The listing builds one solid part. Answer for the finished solid, in the listing's coordinates (mm). Face numbers are marked on the shaded views. A direction names the side the tool comes from. Give positions to 0.01 mm unless a question says otherwise; leave off trailing zeros. Write each loop counter-clockwise with the first axis right and the second up, starting at its lowest first coordinate (ties: lowest second). Pieces come first, ordered by that corner, then holes. Notation, with made-up numbers: (33, 1) -> (43, 1) arc R27 ccw to (43, 17) -> close; hole circle Ø8 at (-15, 76). An arc over 180 degrees is marked (long way). Write each question's results on one line, items separated by ' | '. Start each with the question number.
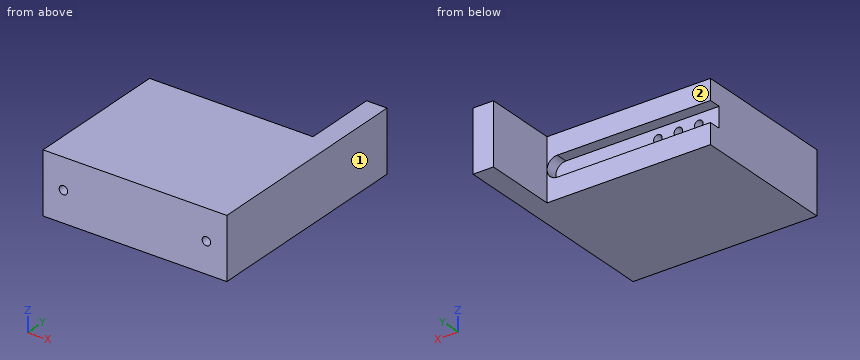
Autodesk Inventor part; units mm, degrees
ref_plane "YZ Plane" through (0, 0, 0) normal (1, 0, 0) x (0, 1, 0)
ref_plane "XZ Plane" through (0, 0, 0) normal (0, 1, 0) x (-1, 0, 0)
ref_plane "XY Plane" through (0, 0, 0) normal (0, 0, 1) x (1, 0, 0)
sketch "Sketch1" plane through (0, 0, 0) normal (0, 0, 1) x (1, 0, 0)
  line L0 (0, 0) -> (57.15, 0)
  line L1 (57.15, 0) -> (57.15, 68.2498)
  line L2 (57.15, 68.2498) -> (0, 68.2498)
  line L3 (0, 68.2498) -> (0, 0)
  line L4 (0, 68.2498) -> (50.8, 68.2498)
  line L5 (50.8, 68.2498) -> (50.8, 45.3898)
  line L6 (50.8, 45.3898) -> (0, 45.3898)
  line L7 (0, 45.3898) -> (0, 68.2498)
  dimension "d0" = 57.15
  dimension "d1" = 68.2498
  dimension "d2" = 50.8
  dimension "d3" = 22.86
extrude "Extrusion1" add sketch "Sketch1" along normal blind 19.05 contours L3 L6 L5 L2 L1 L0
sketch "Sketch2" plane through (0, 45.3898, 0) normal (0, 1, 0) x (1, 0, 0)
  line L0 (0, 0) -> (0, -19.05)
  line L1 (0, -6.35) -> (47.625, -6.35)
  line L2 (47.625, -6.35) -> (47.625, -12.7)
  line L3 (47.625, -12.7) -> (0, -12.7)
  line L4 (0, -12.7) -> (0, -6.35)
  line L5 (0, 0) -> (50.8, 0)
  circle A0 centre (47.625, -9.525) radius 3.175
  dimension "d6" = 47.625
  dimension "d7" = 6.35
  dimension "d8" = 6.35
extrude "Extrusion2" cut sketch "Sketch2" against normal blind 3.7084
sketch "Sketch3" plane through (0, 41.6814, 0) normal (0, 1, 0) x (1, 0, 0)
  line L0 (47.625, -12.7) -> (0, -12.7)
  line L1 (0, -6.35) -> (47.625, -6.35)
  line L2 (0, -12.7) -> (0, -6.35)
  point P0 (0, 0)
  point P1 (6.35, -9.525)
  point P2 (12.7, -9.525)
  point P3 (19.05, -9.525)
  dimension "d11" = 6.35
  dimension "d12" = 3.175
  dimension "d13" = 3.175
  dimension "d14" = 3.175
  dimension "d15" = 6.35
  dimension "d16" = 12.7
  dimension "d17" = 19.05
sketch "Sketch4" plane through (0, 0, 0) normal (0, -1, 0) x (1, 0, 0)
  line L0 (0, 0) -> (57.15, 0)
  line L1 (0, 19.05) -> (57.15, 19.05)
  line L2 (0, 0) -> (0, 19.05)
  line L3 (57.15, 0) -> (57.15, 19.05)
  point P0 (6.35, 9.525)
  point P1 (50.8, 9.525)
  dimension "d18" = 19.05
  dimension "d19" = 9.525
  dimension "d20" = 9.525
  dimension "d21" = 6.35
  dimension "d22" = 6.35
hole "Hole1" at (50.8, 0, 9.525) at (6.35, 0, 9.525) direction (0, 1, 0) diameter 2.6416 depth 7.112 tip angle 118
hole "Hole2" at (6.35, 41.6814, 9.525) at (12.7, 41.6814, 9.525) at (19.05, 41.6814, 9.525) direction (0, -1, 0) diameter 2.6416 depth 7.112 tip angle 118
equation "\"d8\" = d7"
properties part number "Spring block"
1. Section A-A (x = 35.5) is taken. Write down the section's boundary in (y, z), then the cut area to 3 significant figures.
2. Section C-C (y = 54) is taken. Write down the section's boundary in (x, z).
3. Consider probe 1 along Z at (x, y) = (6.35, 5); probe 2 along Y at (x, z) = (36, 2.25); probe 3 along Z at (x, y) = (38, 45). Determine where each line is inside the solid, lowest interval first. Write a range as [from, to].
4. Section B-B (z = 15) is taken. Write down the section's boundary in (x, y), then the cut area to 3 significant figures.
5. A tool of negligible diameter and unlimited length cuts with its end or side. For the marked faces 1 and 2, from which of +Z, -Z, +X, -X, +Y, -Y can it reach the whole face along a straight path? Write none if from no direction.
6. Each of these flat-tipped pins is pushed along its axis until it touches: pin 1 Ø5 at (x, z) = (22.5, 16.5) entering from +Y; pin 2 Ø2 at (x, z) = (50.8, 9.525) entering from -Y; pin 3 Ø1.6 at (x, z) = (19.05, 9.525) entering from +Y. Where does it stop, or does it pass through?
Results:
1) outline: (0, 0) -> (45.39, 0) -> (45.39, 6.35) -> (41.68, 6.35) -> (41.68, 12.7) -> (45.39, 12.7) -> (45.39, 19.05) -> (0, 19.05) -> close | area: 841 mm²
2) outline: (50.8, 0) -> (57.15, 0) -> (57.15, 19.05) -> (50.8, 19.05) -> close
3) probe 1: z = [0, 8.2], [10.85, 19.05] | probe 2: y = [0, 45.39] | probe 3: z = [0, 6.35], [12.7, 19.05]
4) outline: (0, 0) -> (57.15, 0) -> (57.15, 68.25) -> (50.8, 68.25) -> (50.8, 45.39) -> (0, 45.39) -> close | area: 2,740 mm²
5) face 1: +Z, -Z, +X, +Y, -Y | face 2: +Z, -Z, -X, +Y
6) pin 1: stops at y = 45.39 | pin 2: stops at y = 7.3 | pin 3: stops at y = 34.26
